Can you work these out from the model? Positions are in its coordinate system, mm. A direction names the side the tool comes from. Round coordinates to 2 decimals unless told otherwise and drop trailing zeros. Loops run counter-clockwise (first coordinate to the right, second up) from the corner with the lowest first, then second, coordinate; pieces in that order, holes last.
(1) I want a section at C-C on z = 148. Write out the boundary of the cut face in (x, y), plus the area to 3 significant figures.
(2) I want a section at A-A on x = 176.5. Write out the boundary of the cut face in (y, z).
(3) I want a section at B-B on z = 53.5. Write out the boundary of the cut face in (x, y), plus the area to 3 significant figures.
(4) If I drill on line 1 along Z through (x, y) = (95, 1.4); line 2 along Z through (x, y) = (114.5, 1.8); line 3 along X through (y, z) = (6.75, 58.5), over which ranges is the centre line in solid material (lowest first)?
(5) I want a section at D-D on x = 39. Write out the boundary of the cut face in (y, z).
(6) Which directions (+Z, -Z, +X, -X, +Y, -Y) give clear straight access to the entire face, cutting with the end or side of a thin tool? Please do faces 4 (the face through (180, 2, 15)), 5 (the face through (67, 6, 15)), 6 (the face through (10, 2, 15)).
(7) Thinking about a two-plate mould opening in Z: for faces 1 (the face through (123, 6, 40)), 2 (the face through (123, 6.4, 27.6)), 3 (the face through (120, 6, 27)), which applies, released by +Z, released by -Z, zero draft, split by the parting line, or undercut?
(8) Will these pins go through, and if not, where does the flat tip stop? pin 1 Ø5 at (x, z) = (62.5, 51) entering from +Y; pin 2 Ø5 at (y, z) = (3, 146.5) entering from +X; pin 3 Ø2 at (x, y) = (10, 2) entering from +Z; pin 4 Ø1.9 at (x, z) = (27.5, 12) entering from -Y.
Autodesk Inventor part; units mm, degrees
ref_plane "YZ Plane" through (0, 0, 0) normal (1, 0, 0) x (0, 1, 0)
ref_plane "XZ Plane" through (0, 0, 0) normal (0, 1, 0) x (-1, 0, 0)
ref_plane "XY Plane" through (0, 0, 0) normal (0, 0, 1) x (1, 0, 0)
sketch "Sketch1" plane through (0, 0, 0) normal (0, 1, 0) x (-1, 0, 0)
  line L0 (0, 0) -> (-190, 0)
  line L1 (0, 0) -> (0, 15)
  line L2 (-170, 15) -> (-170, 40)
  line L3 (-20, 40) -> (-20, 15)
  line L4 (-20, 15) -> (0, 15)
  line L5 (-20, 40) -> (0, 40)
  line L6 (-170, 15) -> (-190, 15)
  line L7 (-170, 40) -> (-190, 40)
  line L8 (0, 15) -> (0, 0)
  line L9 (-190, 0) -> (-190, 15)
  line L10 (-95, 0) -> (-95, 180)
  line L11 (0, 40) -> (0, 90)
  line L12 (-190, 40) -> (-190, 90)
  line L13 (-95, 180) -> (-75, 180)
  line L14 (-75, 180) -> (0, 90)
  line L15 (-95, 180) -> (-115, 180)
  line L16 (-115, 180) -> (-190, 90)
  dimension "d1" = 190
  dimension "d37" = 180
  dimension "d38" = 50
  dimension "d39" = 20
  dimension "d40" = 20
extrude "Extrusion1" add sketch "Sketch1" along normal blind 4
sketch "Sketch5" plane through (0, 4, 0) normal (0, 1, 0) x (1, 0, 0)
  circle A0 centre (27.5, -12) radius 1.55
  circle A1 centre (27.5, -43) radius 1.55
  circle A2 centre (162.5, -43) radius 1.55
  circle A3 centre (162.5, -12) radius 1.55
  point P0 (0, 0)
extrude "Extrusion2" cut sketch "Sketch5" against normal blind 10
sketch "Sketch6" plane through (0, 4, 0) normal (0, 1, 0) x (1, 0, 0)
  line L0 (20, -15) -> (20, -40)
  line L1 (70, -15) -> (70, -40)
  line L2 (70, -40) -> (64, -40)
  line L3 (64, -40) -> (64, -15)
  line L4 (64, -15) -> (70, -15)
  line L5 (190, 0) -> (0, 0)
  line L6 (120, -15) -> (120, -40)
  line L7 (120, -40) -> (126, -40)
  line L8 (126, -40) -> (126, -15)
  line L9 (126, -15) -> (120, -15)
  dimension "d24" = 6
extrude "Extrusion3" add sketch "Sketch6" along normal blind 5
sketch "Sketch7" plane through (126, 4, 40) normal (1, 0, 0) x (0, 0, -1)
  line L0 (0, 0) -> (25, 0)
  arc A0 (4.8685, 5) -> (20.1315, 5) centre (12.5, 14.9) ccw
  line L1 (0, 5) -> (25, 5)
  line L2 (4.8685, 5) -> (20.1315, 5)
  point P0 (40, -4)
  point P1 (4.8685, 5)
extrude "Extrusion4" cut sketch "Sketch7" against normal blind 10
sketch "Sketch8" plane through (70, 4, 40) normal (1, 0, 0) x (0, 0, -1)
  line L0 (0, 0) -> (25, 0)
  arc A0 (4.8685, 5) -> (20.1315, 5) centre (12.5, 14.9) ccw
  line L1 (25, 5) -> (0, 5)
  arc A1 (4.8685, 5) -> (20.1315, 5) centre (12.5, 14.9) ccw
  line L2 (20.1315, 5) -> (4.8685, 5)
  point P0 (40, -4)
  point P1 (4.8685, 5)
extrude "Extrusion5" cut sketch "Sketch8" against normal blind 10
sketch "Sketch9" plane through (0, 4, 0) normal (0, 1, 0) x (1, 0, 0)
  circle A0 centre (67, -46.379) radius 1.55
  circle A1 centre (123, -46.379) radius 1.55
  circle A2 centre (123, -8.621) radius 1.55
  circle A3 centre (67, -8.621) radius 1.55
  point P0 (0, 0)
extrude "Extrusion6" cut sketch "Sketch9" against normal blind 10
sketch "Sketch10" plane through (0, 4, 0) normal (0, 1, 0) x (1, 0, 0)
  circle A0 centre (67, -46.379) radius 1.55
  circle A1 centre (123, -46.379) radius 1.55
  line L0 (46.35, -50) -> (43.95, -50)
  line L1 (43.95, -50) -> (43.95, -130.85)
  line L2 (43.95, -130.85) -> (46.35, -130.85)
  line L3 (46.35, -130.85) -> (46.35, -50)
  line L4 (146.05, -50) -> (143.65, -50)
  line L5 (143.65, -50) -> (143.65, -130.85)
  line L6 (143.65, -130.85) -> (146.05, -130.85)
  line L7 (146.05, -130.85) -> (146.05, -50)
  point P0 (0, 0)
  dimension "d89" = 2.4
  dimension "d90" = 80.85
  dimension "d92" = 2.4
  dimension "d93" = 80.85
  dimension "d94" = 97.3
extrude "Extrusion7" add sketch "Sketch10" along normal blind 4 contours L3 L2 L1 L0 | L7 L6 L5 L4
sketch "Sketch14" plane through (0, 4, 0) normal (0, 1, 0) x (1, 0, 0)
  line L0 (190, 0) -> (0, 0)
  line L1 (0, 0) -> (0, -7.5)
  line L2 (0, 0) -> (0, -15)
  line L3 (0, -90) -> (75, -180)
  circle A0 centre (7.5, -7.5) radius 1.55
  circle A1 centre (7.5, -90) radius 1.55
  line L4 (75, -180) -> (115, -180)
  circle A2 centre (182.5, -7.5) radius 1.55
  circle A3 centre (182.5, -90) radius 1.55
  circle A4 centre (95, -172.5) radius 1.55
  dimension "d68" = 7.5
  dimension "d71" = 3.1
  dimension "d72" = 3.1
  dimension "d74" = 3.1
extrude "Extrusion10" cut sketch "Sketch14" against normal blind 10
sketch "Sketch15" plane through (0, 4, 0) normal (0, 1, 0) x (1, 0, 0)
  circle A0 centre (140.65, -44.3) radius 1.55
  circle A1 centre (140.65, -136.55) radius 1.55
  circle A2 centre (49.35, -136.55) radius 1.55
  circle A3 centre (49.35, -44.3) radius 1.55
  point P0 (0, 0)
extrude "Extrusion11" cut sketch "Sketch15" against normal blind 10
sketch "Sketch16" plane through (0, 4, 0) normal (0, 1, 0) x (1, 0, 0)
  circle A0 centre (167.6524, -65.2346) radius 1.5
  circle A1 centre (151.6574, -95.6346) radius 1.5
  point P0 (0, 0)
extrude "Extrusion12" cut sketch "Sketch16" against normal blind 10
sketch "Sketch17" plane through (0, 4, 0) normal (0, 1, 0) x (1, 0, 0)
  circle A0 centre (95, -152.3364) radius 14.25
  line L0 (75, -180) -> (115, -180)
  point P0 (0, 0)
  dimension "d101" = 28.5
  dimension "d112" = 27.6636
extrude "Extrusion13" cut sketch "Sketch17" against normal through all
sketch "Sketch19" plane through (0, 4, 0) normal (0, 1, 0) x (1, 0, 0)
  circle A0 centre (95, -152.3364) radius 14.25
  circle A1 centre (114.5, -152.3364) radius 1.55
  circle A2 centre (75.5, -152.3364) radius 1.55
  point P0 (0, 0)
  dimension "d108" = 3.1
  dimension "d109" = 3.1
extrude "Extrusion14" cut sketch "Sketch19" against normal blind 5 contours A1 | A2
properties part number "bp_v2" material "PET Plastic"
Filled sheet:
1. outline: (48.33, 0) - (81.43, 0) - (81.43, 4) - (48.33, 4) - close; (108.57, 0) - (141.67, 0) - (141.67, 4) - (108.57, 4) - close
1. area: 265 mm2
2. outline: (0, 0) - (4, 0) - (4, 15) - (0, 15) - close; (0, 40) - (4, 40) - (4, 106.2) - (0, 106.2) - close
3. outline: (0, 0) - (190, 0) - (190, 4) - (146.05, 4) - (146.05, 8) - (143.65, 8) - (143.65, 4) - (46.35, 4) - (46.35, 8) - (43.95, 8) - (43.95, 4) - (0, 4) - close
3. area: 779 mm2
4. line 1: z = 0 to 138.09, 166.59 to 170.95, 174.05 to 180
4. line 2: z = 0 to 150.79, 153.89 to 180
4. line 3: x = 43.95 to 46.35, 143.65 to 146.05
5. outline: (0, 0) - (4, 0) - (4, 136.8) - (0, 136.8) - close
6. face 4: +X, +Y, -Y
6. face 5: -Z, +X, -X, +Y
6. face 6: -X, +Y, -Y
7. face 1: released by +Z
7. face 2: undercut
7. face 3: zero draft
8. pin 1: stops at y = 4
8. pin 2: stops at x = 145
8. pin 3: stops at z = 103.2
8. pin 4: passes through
